Model file for the job. Use its own axes, mm. Give positions to 0.01 mm unless a question says otherwise; leave off trailing zeros. Write each loop counter-clockwise with the first axis right and the second up, starting at its lowest first coordinate (ties: lowest second). Pieces come first, ordered by that corner, then holes. Notation, with made-up numbers: M -9,-10 L 22,-10 A31 ccw 22,26 Z; hole C -35.75,-31 d10. An arc over 180 degrees is marked long. Answer as a JSON object with one key per item and string values. Group by question number.
```python
from build123d import *

# Parameters (mm, degrees)
BASPROSKE_W           = 5.5
BASPROSKE_H           = 44
TOOTHCUT_DEPTH        = 63.467991804
TEETHCUTS_COUNT       = 20
TEETHCUTS_ANGLE       = 342
BORSKE_R              = 0.5
BORE_DEPTH            = 50.0000508
CORTAR_EXTRUIR1_DEPTH = 5.5


with BuildPart() as part:
    # BasProSke → Base-Revolve (revolve)
    with BuildSketch(Plane(origin=(0, 0, 0), x_dir=(1, 0, 0), z_dir=(0, 1, 0)), mode=Mode.PRIVATE) as base_revolve_sk:
        with Locations((2.75, 22)):
            Rectangle(BASPROSKE_W, BASPROSKE_H)
    revolve(base_revolve_sk.sketch.rotate(Axis((-10, 0, 0), (1, 0, 0)), 180), axis=Axis((-10, 0, 0), (1, 0, 0)))

    # TooCutSke → ToothCut (cut, through all)
    with BuildSketch(Plane(origin=(0, 0, 0), x_dir=(0, 0, -1), z_dir=(1, 0, 0))):
        with BuildLine():
            ThreePointArc((1.961730392, 34.943978235), (0, 34.999), (-1.961730392, 34.943978235))
            ThreePointArc((-1.961730392, 34.943978235), (-3.235659864, 39.585086827), (-5.832115241, 43.637395396))
            ThreePointArc((-5.832115241, 43.637395396), (0, 44.0254), (5.832115241, 43.637395396))
            ThreePointArc((5.832115241, 43.637395396), (3.235659864, 39.585086827), (1.961730392, 34.943978235))
        make_face()
    toothcut = extrude(amount=TOOTHCUT_DEPTH, mode=Mode.SUBTRACT)

    # TeethCuts: ToothCut ×20 about axis
    teethcuts_axis = Axis((-10, 0, 0), (1, 0, 0))
    for i in range(1, TEETHCUTS_COUNT):
        add(toothcut.rotate(teethcuts_axis, i * TEETHCUTS_ANGLE / (TEETHCUTS_COUNT - 1)), mode=Mode.SUBTRACT)

    # BorSke → Bore (cut, symmetric)
    with BuildSketch(Plane(origin=(0, 0, 0), x_dir=(0, 0, -1), z_dir=(1, 0, 0))):
        with Locations(Location((0, 0, 0), (0, 0, 180))):
            Circle(BORSKE_R)
    extrude(amount=BORE_DEPTH, both=True, mode=Mode.SUBTRACT)

    # Croquis1 → Cortar-Extruir1 (cut)
    with BuildSketch(Plane(origin=(5.5, 0, 0), x_dir=(0, 0, -1), z_dir=(1, 0, 0))):
        with BuildLine():
            Line((-3.51323213, 1.435), (3.51323213, 1.435))
            ThreePointArc((3.51323213, 1.435), (0, -3.795), (-3.51323213, 1.435))
        make_face()
    extrude(amount=-CORTAR_EXTRUIR1_DEPTH, mode=Mode.SUBTRACT)


solid = part.part
```
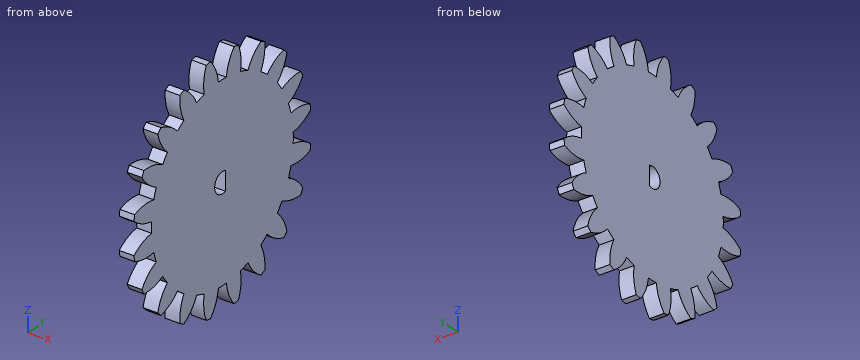
Q1. Drop flat-ended pins along their axis: P1, Ø12, axis at y = 9.5, z = -13, coming from the -X side; P2, Ø1.5, axis at x = 3.5, z = 27.5, coming from the +Y side; P3, Ø1, axis at x = 3.5, z = -10, coming from the -Y side (3 decimals); P4, Ø1.5, axis at x = 4, z = -29, coming from the -Y side. Give the stop position or say it passes through.
Q2. Slice it at B-B, the plane y = 0. Write the cut outline in (x, z) (3 decimals), then the cut area to 3 significant figures.
Q3. Slice it at D-D, the plane z = 37.5. Write the cut outline in (x, y).
Q4. Wall check: L1, parallel to Z at x = 2.05, y = 34; L2, parallel to Z at x = 1.1, y = 0 (3 decimals); L3, parallel to Z at x = 4.85, y = -37. Give the ranges that are in metal, low to high.
Q5. Slice it at A-A, the plane z = 0. Write the cut outline in (x, y) (3 decimals).
Q6. Slice it at C-C, the plane y = 36. Write the cut outline in (x, z), then the cut area to 3 significant figures.
Solved:
{
 "1": {"P1": "stops at x = 0", "P2": "stops at y = 31.24", "P3": "stops at y = -33.685", "P4": "stops at y = -31.72"},
 "2": {"outline": "M 0,-34.999 L 5.5,-34.999 L 5.5,-3.795 L 0,-3.795 Z; M 0,3.795 L 5.5,3.795 L 5.5,34.999 L 0,34.999 Z", "area": "343 mm²"},
 "3": {"outline": "M 0,-21 L 5.5,-21 L 5.5,-16.14 L 0,-16.14 Z; M 0,-9.23 L 5.5,-9.23 L 5.5,-2.48 L 0,-2.48 Z; M 0,2.48 L 5.5,2.48 L 5.5,9.23 L 0,9.23 Z; M 0,16.14 L 5.5,16.14 L 5.5,21 L 0,21 Z"},
 "4": {"L1": "z = -20.67 to -13.38, -8.96 to 8.96, 13.38 to 20.67", "L2": "z = -34.999 to -3.795, 3.795 to 34.999", "L3": "z = -21 to -15.64, -9.24 to -2.34, 2.34 to 9.24, 15.64 to 21"},
 "5": {"outline": "M 0,-34.999 L 5.5,-34.999 L 5.5,-3.795 L 0,-3.795 Z; M 0,1.435 L 5.5,1.435 L 5.5,34.999 L 0,34.999 Z"},
 "6": {"outline": "M 0,-20.95 L 5.5,-20.95 L 5.5,-14.76 L 0,-14.76 Z; M 0,-9.21 L 5.5,-9.21 L 5.5,-2.12 L 0,-2.12 Z; M 0,2.12 L 5.5,2.12 L 5.5,9.21 L 0,9.21 Z; M 0,14.76 L 5.5,14.76 L 5.5,20.95 L 0,20.95 Z", "area": "146 mm²"}
}
